Model file for the job. Use its own axes, mm. A direction names the side the tool comes from. Give positions to 0.01 mm unless a question says otherwise; leave off trailing zeros. Write each loop counter-clockwise with the first axis right and the second up, starting at its lowest first coordinate (ties: lowest second). Pieces come first, ordered by that corner, then holes.
```python
from build123d import *

# Parameters (mm, degrees)
BOSS_EXTRUDE1_DEPTH      = 4.572
BOSS_EXTRUDE2_DEPTH      = 0.762
BOSS_EXTRUDE2_DEPTH_BACK = 5.334
SKETCH2_R                = 2.869299529
SKETCH3_R                = 1.397
CUT_EXTRUDE1_DEPTH       = 44.588683524


with BuildPart() as part:
    # Sketch1 → Boss-Extrude1 (new body)
    with BuildSketch(Plane(origin=(0, 0, 0), x_dir=(1, 0, 0), z_dir=(0, 1, 0))):
        with BuildLine():
            Line((0, 23.945183489), (16.621899459, -21.723109944))
            ThreePointArc((16.621899459, -21.723109944), (18.758742816, -22.611950557), (20.0669487, -24.521069341))
            Line((20.0669487, -24.521069341), (11.850067084, -27.178766186))
            Line((11.850067084, -27.178766186), (5.178997556, -8.850153293))
            ThreePointArc((5.178997556, -8.850153293), (2.119691783, -6.751008186), (0.941519753, -3.232816511))
            ThreePointArc((0.941519753, -3.232816511), (-4.609142435, -0.625246171), (-10.668, 0.323183489))
            Line((-10.668, 0.323183489), (-28.650367288, 0.323183489))
            ThreePointArc((-28.650367288, 0.323183489), (-28.941106082, 0.241834206), (-29.19191304, 0.073778793))
            ThreePointArc((-29.19191304, 0.073778793), (-33.527942998, 1.06904003), (-29.206401998, 2.125441522))
            ThreePointArc((-29.206401998, 2.125441522), (-28.965026953, 1.944099747), (-28.679100404, 1.847183489))
            Line((-28.679100404, 1.847183489), (-0.508, 1.847183489))
            ThreePointArc((-0.508, 1.847183489), (0, 2.355183489), (-0.508, 2.863183489))
            Line((-0.508, 2.863183489), (-15.24, 2.863183489))
            ThreePointArc((-15.24, 2.863183489), (-11.9126, 13.404183489), (-15.24, 23.945183489))
            Line((-15.24, 23.945183489), (0, 23.945183489))
        make_face()
    extrude(amount=BOSS_EXTRUDE1_DEPTH)

    # Sketch2 → Boss-Extrude2 (add, two sides: drawn at the far end of the back side and taken through both)
    with BuildSketch(Plane(origin=(0, 4.572, 0), x_dir=(1, 0, 0), z_dir=(0, 1, 0)).offset(-BOSS_EXTRUDE2_DEPTH_BACK)):
        with Locations(Location((6.807711808, -3.148121568, 0), (0, 0, 270))):
            Circle(SKETCH2_R)
    extrude(amount=BOSS_EXTRUDE2_DEPTH + BOSS_EXTRUDE2_DEPTH_BACK)

    # Sketch3 → Cut-Extrude1 (cut, through all)
    with BuildSketch(Plane(origin=(0, 5.334, 0), x_dir=(1, 0, 0), z_dir=(0, 1, 0))):
        with Locations(Location((6.807711808, -3.148121568, 0), (0, 0, 270))):
            Circle(SKETCH3_R)
    extrude(amount=-CUT_EXTRUDE1_DEPTH, mode=Mode.SUBTRACT)


solid = part.part
```
1. Slice it at B-B, the plane y = 3.75. Write the cut outline in (x, z).
Calculated:
outline: (-29.21, -2.13) arc R0.95 cw to (-28.68, -1.85) - (-0.51, -1.85) arc R0.51 cw to (-0.51, -2.86) - (-15.24, -2.86) arc R18.36 cw to (-15.24, -23.95) - (0, -23.95) - (16.62, 21.72) arc R4.08 ccw to (20.07, 24.52) - (11.85, 27.18) - (5.18, 8.85) arc R5.84 ccw to (0.94, 3.23) arc R21.67 cw to (-10.67, -0.32) - (-28.65, -0.32) arc R0.95 cw to (-29.19, -0.07) arc R2.29 ccw (long way) to start; hole circle Ø2.79 at (6.81, 3.15)
2. Which spindle directions (+Z, -Z, +X, -X, +Y, -Y) get a long thin tool onto all of the face, cutting with end or side? Do faces 4 (the cylindrical face through (18.73, 2.25, 22.59)), 5 (the flat face through (-15, 2, -1.847)), 6 (the cylindrical face through (5.06, -0.39, 0.87)), 7 (the flat face through (-20, 2, -0.323)). Say none if no direction does.
Calculated:
face 4: -Z, +X, +Y, -Y
face 5: +Y, -Y
face 6: -Y
face 7: +Z, +Y, -Y
3. Pull direction Z, two halves, no side cores. Call faces 1 (the cylindrical face through (5.06, 4.95, 0.87)), 2 (the cylindrical face through (-4.53, 2.25, 0.65)), 3 (the flat face through (-8, 2, -2.863)): +Z half, -Z half, draft (parallel to the pull), parting line (faces both ways), or undercut.
Calculated:
face 1: parting line
face 2: +Z half
face 3: undercut
4. Slice it at C-C, the plane x = -22.5. Write the cut outline in (y, z), and give its area (3 significant figures).
Calculated:
outline: (0, -1.85) - (4.57, -1.85) - (4.57, -0.32) - (0, -0.32) - close
area: 6.97 mm2
5. Pin check, flat tips, straight feed: P1, Ø2.5, axis at x = -8.5, y = 1.5, coming from the +Z side; P2, Ø1.7, axis at x = 6.81, z = 3.15, coming from the +Y side; P3, Ø2.5, axis at x = -18.5, y = 1, coming from the +Z side; P4, Ø1.5, axis at y = 1, z = 12, coming from the -X side. Stop position of each tip, or through.
Calculated:
P1: stops at z = -0.01
P2: passes through
P3: stops at z = -0.32
P4: stops at x = 6.05
6. Slice it at A-A, the plane x = -5.5. Write the cut outline in (y, z), and give its area (3 significant figures).
Calculated:
outline: (0, -23.95) - (4.57, -23.95) - (4.57, -2.86) - (0, -2.86) - close; (0, -1.85) - (4.57, -1.85) - (4.57, 0.37) - (0, 0.37) - close
area: 107 mm2
7. Slice it at D-D, the plane z = -13. Write the cut outline in (x, y).
Calculated:
outline: (-11.92, 0) - (3.98, 0) - (3.98, 4.57) - (-11.92, 4.57) - close
8. Probe probe 1 along Y at (x, z) = (-5, -10.5); probe 2 along X at (y, z) = (1.5, 24); probe 3 along Z at (x, y) = (-6, 3.75). List the from-to ranges inside material, lowest first.
Calculated:
probe 1: y = 0 to 4.57
probe 2: x = 10.69 to 19.86
probe 3: z = -23.95 to -2.86, -1.85 to 0.25
